from build123d import *

# Parameters (mm, degrees)
F1_DEPTH       = 35
F1_DEPTH_BACK  = 35
F3_DEPTH       = 49
F4_R           = 1.99
F5_R           = 3.9
F6_DEPTH       = 25
F8_DEPTH       = 2.5
F10_DEPTH      = 11.5
F10_DEPTH_BACK = 11.5
F11_R          = 4.99999


# Not quite as in the source:
# - a fillet or chamfer is up to 0.001 mm smaller than in the source, because OpenCascade refuses the exact size


with BuildPart() as f1:
    # F0 (on Right) → F1 (new body, two sides)
    with BuildSketch(Plane.YZ) as f1_sk:
        Polygon((15, 0), (0, 0), (0, 6.5), (10, 6.5), (10, 11.5), (-5, 11.5), (-5, -5), (-5, -42.5), (0, -42.5), (0, -5), (15, -5), align=None)
    extrude(amount=F1_DEPTH)
    extrude(f1_sk.sketch, amount=-F1_DEPTH_BACK)

    # F2 (on face) → F3 (join, through all)
    with BuildSketch(Plane(origin=(0, 0, 6.5), x_dir=(1, 0, 0), z_dir=(0, 0, -1))):
        Polygon((7.5, 18), (7.5, 5), (11.5, 5), (11.5, 22), (0, 22), (-11.5, 22), (-11.5, 5), (-7.5, 5), (-7.5, 18), (0, 18), align=None)
    extrude(amount=F3_DEPTH)

    # F4
    f4_edges = [f1.edges().sort_by_distance(p)[0] for p in [
        (11.5, -13.5, 6.5),
        (7.5, -11.5, 6.5),
        (-7.5, -11.5, 6.5),
        (0, -18, 6.5),
        (0, -22, 6.5),
        (-11.5, -13.5, 6.5),
        (-11.5, -22, -18),
        (11.5, -22, -18),
    ]]
    fillet(f4_edges, radius=F4_R)

    # F5 (on face) → F6 (cut)
    with BuildSketch(Plane.XZ.offset(5)):
        with Locations((23.5, -11)):
            Circle(F5_R)
        with Locations((23.5, -31)):
            Circle(F5_R)
        with Locations((-23.5, -11)):
            Circle(F5_R)
        with Locations((-23.5, -31)):
            Circle(F5_R)
    extrude(amount=-F6_DEPTH, mode=Mode.SUBTRACT)

    # F7 (on face) → F8 (join)
    with BuildSketch(Plane(origin=(0, 0, -42.5), x_dir=(1, 0, 0), z_dir=(0, 0, -1))):
        Polygon((1.5, 18), (0, 18), (-1.5, 18), (-1.5, 13), (-7.5, 13), (-7.5, 11.5), (-7.5, 10), (-1.5, 10), (-1.5, 5), (0, 5), (1.5, 5), (1.5, 10), (7.5, 10), (7.5, 11.5), (7.5, 13), (1.5, 13), align=None)
    extrude(amount=-F8_DEPTH)

    # F9 (on Right) → F10 (join, two sides)
    with BuildSketch(Plane.YZ) as f10_sk:
        Polygon((0, -5), (0, -42.5), (15, -5), align=None)
    extrude(amount=-F10_DEPTH)
    extrude(f10_sk.sketch, amount=F10_DEPTH_BACK)

    # F11 (radius 5 in the source; OpenCascade refuses exactly that, so slightly less here)
    f11_edges = [f1.edges().sort_by_distance(p)[0] for p in [
        (-23.25, -5, -42.5),
        (23.25, -5, -42.5),
        (0, 10, 11.5),
        (35, 2.5, 11.5),
        (-35, 2.5, 11.5),
        (0, -5, 11.5),
        (-35, -5, -15.5),
        (35, -5, -15.5),
        (11.5, 7.5, -23.75),
        (-11.5, 7.5, -23.75),
        (35, 15, -2.5),
        (-35, 15, -2.5),
    ]]
    fillet(f11_edges, radius=F11_R)


solid = f1.part
Can you work these out from the model? Positions are in its coordinate system, mm. A direction names the side the tool comes from. Coordinates: 2 decimals unless noted, no trailing zeros. Write each loop counter-clockwise with the first axis right and the second up, starting at its lowest first coordinate (ties: lowest second). Pieces come first, ordered by that corner, then holes.
Q1. Which directions (+Z, -Z, +X, -X, +Y, -Y) give clear straight access to the entire face, cutting with the end or side of a thin tool? Please do faces 1 (the face through (5, -13, -41)), 2 (the face through (0, -12, -40)), 3 (the face through (11.5, 4, -14)).
Results found:
face 1: +Z, -Z
face 2: +Z
face 3: -Z, +X, +Y
Q2. Imagine slicing it at A-A, the plane y = -6. Count the separate pieces of the cut face and the enclosed holes in it, plus the area to 3 significant figures.
Results found:
separate pieces: 3
enclosed holes: 0
area: 396 mm2
Q3. Imagine slicing it at B-B, the plane z = -3. List the corners of the cut face in (x, y) for me.
Results found:
outline: (-35, 0) arc R5 ccw to (-30, -5) - (-11.5, -5) - (-11.5, -20.01) arc R1.99 ccw to (-9.51, -22) - (9.51, -22) arc R1.99 ccw to (11.5, -20.01) - (11.5, -5) - (30, -5) arc R5 ccw to (35, 0) - (35, 10) arc R5 ccw to (30, 15) - (-30, 15) arc R5 ccw to (-35, 10) - close; hole (-7.5, -18) - (7.5, -18) - (7.5, -5) - (-7.5, -5) - close
Q4. If we mould it in two halves opening along Z, with no side actions, what happens to faces 4 (the face through (0, 8, 0)), 5 (the face through (1.5, -15, -41)), 6 (the face through (0, 0, 3)), 7 (the face through (-33.57, 3.82, 10))? For each: +Z half, -Z half, draft (parallel to the pull), parting line (faces both ways), or undercut.
Results found:
face 4: undercut
face 5: draft
face 6: undercut
face 7: +Z half
Q5. Please list where these lines run through material, in increasing order: L1, parallel to X at y = -13.5, z = -14; L2, parallel to Z at x = 23.5, y = -2.85; L3, parallel to Z at x = 23.5, y = -2.75.
Results found:
L1: x = -11.5 to -7.5, 7.5 to 11.5
L2: z = -41.61 to -34.9, -27.1 to -14.9, -7.1 to 10.61
L3: z = -41.68 to -34.9, -27.1 to -14.9, -7.1 to 10.68
Q6. For P1, Ø10, axis at y = -8, z = -11.5, coming from the +X side; P2, Ø12, axis at x = -2.5, z = -13, coming from the +Y side; P3, Ø4.5, axis at x = 4, y = -11, coming from the +Z side; P4, Ø8, axis at y = 3.5, z = 2, coming from the -X side, each with a flat end and sliding along its axis, tell me the tip position at first contact or that it passes through.
Results found:
P1: stops at x = 34
P2: stops at y = 14.2
P3: stops at z = -40
P4: stops at x = -35
